Build history of the part. All positions in model axes, mm. A direction names the side the tool comes from. Give positions to 0.01 mm unless a question says otherwise; leave off trailing zeros. Use a Markdown table: item, result. Add a question column.
```python
from build123d import *

# Parameters (mm, degrees)
BOX007_W               = 100
BOX007_H               = 100
BOX007_DEPTH           = 100
BOX007_PLACEMENT_ANGLE = -45
BOX006_W               = 100
BOX006_H               = 200
BOX006_DEPTH           = 100
BOX006_PLACEMENT_ANGLE = 45
BOX005_W               = 100
BOX005_H               = 100
BOX005_DEPTH           = 100
BOX004_W               = 20
BOX004_H               = 20
BOX004_DEPTH           = 80
BOX003_W               = 20
BOX003_H               = 20
BOX003_DEPTH           = 80
BOX002_W               = 10
BOX002_H               = 25
BOX002_DEPTH           = 35
BOX002_PITCH_ANGLE     = -15
BOX001_W               = 10
BOX001_H               = 25
BOX001_DEPTH           = 35
BOX001_PITCH_ANGLE     = 15
BOX_W                  = 20
BOX_H                  = 25
BOX_DEPTH              = 35
CYLINDER005_R          = 10
CYLINDER005_DEPTH      = 180
CYLINDER005_ROLL_ANGLE = 90
CYLINDER004_R          = 54
CYLINDER004_DEPTH      = 100
CYLINDER003_R          = 59
CYLINDER003_DEPTH      = 10
CYLINDER002_R          = 64
CYLINDER002_DEPTH      = 85
CYLINDER001_R          = 70
CYLINDER001_DEPTH      = 90
CYLINDER_R             = 80
CYLINDER_DEPTH         = 10
FILLET_R               = 3
FILLET001_R            = 5
FILLET002_R            = 5
CUT009_ROLL_ANGLE      = -90
CUT009_PITCH_ANGLE     = 45
CUT009_PLACEMENT_ANGLE = -45


with BuildPart() as cube004:
    # Box007 → Box007 (new body)
    with BuildSketch(Plane.XY):
        with Locations((50, 50)):
            Rectangle(BOX007_W, BOX007_H)
    extrude(amount=BOX007_DEPTH)


with BuildPart() as cube004_1:
    # Box007 placement: moved
    add(cube004.part.rotate(Axis((0, 0, 0), (0, 0, 1)), BOX007_PLACEMENT_ANGLE))


with BuildPart() as cube003:
    # Box006 → Box006 (new body)
    with BuildSketch(Plane.XY):
        with Locations((50, 100)):
            Rectangle(BOX006_W, BOX006_H)
    extrude(amount=BOX006_DEPTH)


with BuildPart() as cube003_1:
    # Box006 placement: moved
    add(cube003.part.moved(Location((71, -71, 0))).rotate(Axis((71, -71, 0), (0, 0, 1)), BOX006_PLACEMENT_ANGLE))


with BuildPart() as cube002:
    # Box005 → Box005 (new body)
    with BuildSketch(Plane(origin=(0, 0, 0), x_dir=(-1, 0, 0), z_dir=(0, 0, 1))):
        with Locations((50, 50)):
            Rectangle(BOX005_W, BOX005_H)
    extrude(amount=BOX005_DEPTH)


with BuildPart() as tab_cut_l:
    # Box004 → Box004 (new body)
    with BuildSketch(Plane(origin=(-83, -10, 20), x_dir=(1, 0, 0), z_dir=(0, 0, 1))):
        with Locations((10, 10)):
            Rectangle(BOX004_W, BOX004_H)
    extrude(amount=BOX004_DEPTH)


with BuildPart() as tab_cut_r:
    # Box003 → Box003 (new body)
    with BuildSketch(Plane(origin=(63, -10, 20), x_dir=(1, 0, 0), z_dir=(0, 0, 1))):
        with Locations((10, 10)):
            Rectangle(BOX003_W, BOX003_H)
    extrude(amount=BOX003_DEPTH)


with BuildPart() as cube001:
    # Box002 → Box002 (new body)
    with BuildSketch(Plane.XY):
        with Locations((5, 12.5)):
            Rectangle(BOX002_W, BOX002_H)
    extrude(amount=BOX002_DEPTH)


with BuildPart() as cube001_1:
    # Box002 pitch: moved
    add(cube001.part.rotate(Axis((0, 0, 0), (0, 1, 0)), BOX002_PITCH_ANGLE))


with BuildPart() as cube001_2:
    # Box002 placement: moved
    add(cube001_1.part.moved(Location((-9.95, 48, 64))))


with BuildPart() as cube:
    # Box001 → Box001 (new body)
    with BuildSketch(Plane.XY):
        with Locations((5, 12.5)):
            Rectangle(BOX001_W, BOX001_H)
    extrude(amount=BOX001_DEPTH)


with BuildPart() as cube_1:
    # Box001 pitch: moved
    add(cube.part.rotate(Axis((0, 0, 0), (0, 1, 0)), BOX001_PITCH_ANGLE))


with BuildPart() as cube_2:
    # Box001 placement: moved
    add(cube_1.part.moved(Location((0, 48, 65))))


with BuildPart() as bearing_slot:
    # Box → Box (new body)
    with BuildSketch(Plane(origin=(-10, 48, 65), x_dir=(1, 0, 0), z_dir=(0, 0, 1))):
        with Locations((10, 12.5)):
            Rectangle(BOX_W, BOX_H)
    extrude(amount=BOX_DEPTH)


with BuildPart() as bearing_holes:
    # Cylinder005 → Cylinder005 (new body)
    with BuildSketch(Plane.XY):
        Circle(CYLINDER005_R)
    extrude(amount=CYLINDER005_DEPTH)


with BuildPart() as bearing_holes_1:
    # Cylinder005 roll: moved
    add(bearing_holes.part.rotate(Axis((0, 0, 0), (1, 0, 0)), CYLINDER005_ROLL_ANGLE))


with BuildPart() as bearing_holes_2:
    # Cylinder005 placement: moved
    add(bearing_holes_1.part.moved(Location((0, 90, 65))))


with BuildPart() as through_hole:
    # Cylinder004 → Cylinder004 (new body)
    with BuildSketch(Plane.XY):
        Circle(CYLINDER004_R)
    extrude(amount=CYLINDER004_DEPTH)


with BuildPart() as inner_lip:
    # Cylinder003 → Cylinder003 (new body)
    with BuildSketch(Plane.XY.offset(80)):
        Circle(CYLINDER003_R)
    extrude(amount=CYLINDER003_DEPTH)


with BuildPart() as inner_hole:
    # Cylinder002 → Cylinder002 (new body)
    with BuildSketch(Plane.XY):
        Circle(CYLINDER002_R)
    extrude(amount=CYLINDER002_DEPTH)


with BuildPart() as body_cylinder:
    # Cylinder001 → Cylinder001 (new body)
    with BuildSketch(Plane.XY.offset(5)):
        Circle(CYLINDER001_R)
    extrude(amount=CYLINDER001_DEPTH)


with BuildPart() as cut010:
    # Cylinder → Cylinder (new body)
    with BuildSketch(Plane.XY):
        Circle(CYLINDER_R)
    extrude(amount=CYLINDER_DEPTH)

    # Fusion: union Body_Cylinder
    add(body_cylinder.part)

    # Cut: cut Inner_Hole
    add(inner_hole.part, mode=Mode.SUBTRACT)

    # Fusion001: union Inner_Lip
    add(inner_lip.part)

    # Cut001: cut Through_Hole
    add(through_hole.part, mode=Mode.SUBTRACT)

    # Fillet
    fillet_edges = [cut010.edges().sort_by_distance(p)[0] for p in [
        (-70, 0, 10),
    ]]
    fillet(fillet_edges, radius=FILLET_R)

    # Fillet001
    fillet001_edges = [cut010.edges().sort_by_distance(p)[0] for p in [
        (-80, 0, 0),
    ]]
    fillet(fillet001_edges, radius=FILLET001_R)

    # Fillet002
    fillet002_edges = [cut010.edges().sort_by_distance(p)[0] for p in [
        (-70, 0, 95),
    ]]
    fillet(fillet002_edges, radius=FILLET002_R)

    # Cut002: cut Bearing_Holes
    add(bearing_holes_2.part, mode=Mode.SUBTRACT)

    # Cut003: cut Bearing_Slot
    add(bearing_slot.part, mode=Mode.SUBTRACT)

    # Cut004: cut Cube
    add(cube_2.part, mode=Mode.SUBTRACT)

    # Cut005: cut Cube001
    add(cube001_2.part, mode=Mode.SUBTRACT)

    # Cut006: cut Tab_Cut_R
    add(tab_cut_r.part, mode=Mode.SUBTRACT)

    # Cut007: cut Tab_Cut_L
    add(tab_cut_l.part, mode=Mode.SUBTRACT)

    # Cut008: cut Cube002
    add(cube002.part, mode=Mode.SUBTRACT)

    # Cut009: cut Cube003
    add(cube003_1.part, mode=Mode.SUBTRACT)


with BuildPart() as cut010_1:
    # Cut009 roll: moved
    add(cut010.part.rotate(Axis((0, 0, 0), (1, 0, 0)), CUT009_ROLL_ANGLE))


with BuildPart() as cut010_2:
    # Cut009 pitch: moved
    add(cut010_1.part.rotate(Axis((0, 0, 0), (0, 1, 0)), CUT009_PITCH_ANGLE))


with BuildPart() as cut010_3:
    # Cut009 placement: moved
    add(cut010_2.part.rotate(Axis((0, 0, 0), (0, 0, 1)), CUT009_PLACEMENT_ANGLE))

    # Cut010: cut Cube004
    add(cube004_1.part, mode=Mode.SUBTRACT)


solid = cut010_3.part
```
(1) Tool access for faces 1 (the face through (21.29, 98.92, 22.75)), 2 (the face through (-42.18, 56.32, 29.46)), 3 (the face through (-21.72, 50.004, 43.547)), 4 (the face through (19.841, 93.296, 20.118)): list every direction of +Z, -Z, +X, -X, +Y, -Y with a clear straight run to the whole face (end or side of a thin tool).
(2) Pin check, flat tips, straight feed: pin 1 Ø2 at (x, z) = (-39.5, 6.5) entering from -Y; pin 2 Ø10 at (y, z) = (79, 25) entering from +X; pin 3 Ø2 at (x, z) = (-19, 45) entering from +Y. Stop position of each tip, or through.
(3) Mould opens along X. For faces 5 (the face through (33.758, 92.195, 41.321)), 6 (the face through (19.68, 96.94, 22.28)), 7 (the face through (-47.1, 57.66, 30.21)) say: released by +X, released by -X, zero draft, split by the parting line, or undercut.
(4) Wall check: probe 1 along X at (y, z) = (52, 42); probe 2 along X at (y, z) = (94, 25); probe 3 along Y at (x, z) = (35, 41). Give the ranges that are in metal, low to high.
Response:
| question | item | result |
|---|---|---|
| 1 | face 1 | none |
| 1 | face 2 | +Z, +Y |
| 1 | face 3 | +Z, +X |
| 1 | face 4 | -Z, -Y |
| 2 | pin 1 | stops at y = 49.53 |
| 2 | pin 2 | stops at x = 1.62 |
| 2 | pin 3 | stops at y = 48.28 |
| 3 | face 5 | released by +X |
| 3 | face 6 | undercut |
| 3 | face 7 | released by -X |
| 4 | probe 1 | x = -44.29 to -37.86, -27.2 to -23.72 |
| 4 | probe 2 | x = 1.53 to 10.68, 19.14 to 26.31 |
| 4 | probe 3 | y = 92.98 to 99.35 |
